```python
from build123d import *

# Parameters (mm, degrees)
SKETCH_1_R             = 16
EXTRUDE_1_DEPTH        = 12
SKETCH_2_R             = 13
EXTRUDE_2_DEPTH        = 2
SKETCH_3_R             = 12.25
EXTRUDE_4_DEPTH        = 11.2
SKETCH_4_R             = 1.5
EXTRUDE_5_DEPTH        = 2
SKETCH_21_W            = 0.599041837
SKETCH_21_H            = 5.051087673
CUT_EXTRUDE_2_DEPTH    = 5
HOLE_WIZARD_M3_1_D     = 2.5
HOLE_WIZARD_M3_1_DEPTH = 7.5
HOLE_WIZARD_M3_1_TIP   = 0.751075774
EXTRUDE_16_DEPTH       = 15


with BuildPart() as part:
    # 草图1 → 凸台-拉伸1 (new body)
    with BuildSketch(Plane.XY):
        Circle(SKETCH_1_R)
    extrude(amount=-EXTRUDE_1_DEPTH)

    # 草图2 → 凸台-拉伸2 (add)
    with BuildSketch(Plane(origin=(0, 0, -12), x_dir=(-1, 0, 0), z_dir=(0, 0, -1))):
        Circle(SKETCH_2_R)
    extrude(amount=EXTRUDE_2_DEPTH)

    # 草图3 → 凸台-拉伸4 (add)
    with BuildSketch(Plane(origin=(0, 0, -14), x_dir=(-1, 0, 0), z_dir=(0, 0, -1))):
        with Locations(Location((0, 0, 0), (0, 0, 180))):
            Circle(SKETCH_3_R)
    extrude(amount=EXTRUDE_4_DEPTH)

    # 草图4 → 凸台-拉伸5 (add)
    # profile 1 of 2: a face of its own
    with BuildSketch(Plane.XY):
        with BuildLine():
            Line((-4, 19.5), (-4, 15.491933385))
            ThreePointArc((-4, 15.491933385), (0, 16), (4, 15.491933385))
            Line((4, 15.491933385), (4, 19.5))
            ThreePointArc((4, 19.5), (0, 23.5), (-4, 19.5))
        make_face()
        with Locations((0, 19.5)):
            Circle(SKETCH_4_R, mode=Mode.SUBTRACT)
    # profile 2 of 2: a face of its own
    with BuildSketch(Plane.XY):
        with BuildLine():
            Line((-4, -15.491933385), (-4, -19.5))
            ThreePointArc((-4, -19.5), (0, -23.5), (4, -19.5))
            Line((4, -19.5), (4, -15.491933385))
            ThreePointArc((4, -15.491933385), (0, -16), (-4, -15.491933385))
        make_face()
        with Locations(Location((0, -19.5, 0), (0, 0, 180))):
            Circle(SKETCH_4_R, mode=Mode.SUBTRACT)
    extrude(amount=-EXTRUDE_5_DEPTH)

    # 草图17 → 旋转1 (revolve)
    with BuildSketch(Plane(origin=(0, 0, 0), x_dir=(1, 0, 0), z_dir=(0, 1, 0)), mode=Mode.PRIVATE) as revolve_1_sk:
        Polygon((8, -10.2), (8, 0), (3.5, 0), (3.5, -1.25), (4, -1.25), (4, -2.7), (5.5, -2.7), (5.5, -10.2), align=None)
    revolve(revolve_1_sk.sketch.rotate(Axis((8, 0, 10.2), (0, 0, -1)), 180), axis=Axis((8, 0, 10.2), (0, 0, -1)))

    # 草图21 → 切除-拉伸2 (cut)
    with BuildSketch(Plane.XY.offset(10.2)):
        with Locations((5.700479082, -0.105298995)):
            Rectangle(SKETCH_21_W, SKETCH_21_H)
        with Locations((10.299520919, -0.105298995)):
            Rectangle(SKETCH_21_W, SKETCH_21_H)
    extrude(amount=-CUT_EXTRUDE_2_DEPTH, mode=Mode.SUBTRACT)

    # M3 螺纹孔1
    with Locations(Plane.XY.offset(10.2)):
        with Locations((8, 0)):
            Hole(HOLE_WIZARD_M3_1_D / 2, depth=HOLE_WIZARD_M3_1_DEPTH)
            with Locations((0, 0, -(HOLE_WIZARD_M3_1_DEPTH + HOLE_WIZARD_M3_1_TIP / 2))):  # 118° drill point
                Cone(0, HOLE_WIZARD_M3_1_D / 2, HOLE_WIZARD_M3_1_TIP, mode=Mode.SUBTRACT)

    # 草图25 → 凸台-拉伸16 (add)
    with BuildSketch(Plane(origin=(0, 0, 0), x_dir=(0, 0, -1), z_dir=(1, 0, 0))):
        with BuildLine():
            Line((24.65972398, 2.283115818), (24.65972398, -2.515790041))
            ThreePointArc((24.65972398, -2.515790041), (23.758111364, -3.417402657), (22.856498748, -2.515790041))
            Line((22.856498748, -2.515790041), (22.856498748, 2.283115818))
            ThreePointArc((22.856498748, 2.283115818), (23.758111364, 3.184728434), (24.65972398, 2.283115818))
        make_face()
    extrude(amount=EXTRUDE_16_DEPTH)


solid = part.part
```
Source: CAD feature listing. Evaluate the final solid. Frame: model axes, mm. A direction names the side the tool comes from. Round coordinates to 2 decimals unless told otherwise and drop trailing zeros. Loops run counter-clockwise (first coordinate to the right, second up) from the corner with the lowest first, then second, coordinate; pieces in that order, holes last.
1. Section query C-C on x = -9. Output: boundary loops of the cut face in (y, z).
2. Mould query, pull axis Z, two halves, no side actions, for faces 4 (the cylindrical face through (0, -21, -1)), 5 (the flat face through (0, 0, 0)), 6 (the cylindrical face through (13.392, 3.185, -23.738)). Classes: released by +Z, released by -Z, zero draft, split by the parting line, or undercut.
3. Contact query for flat-ended pins moving along their axis: pin 1 (0.6 mm diameter, centred on x = 5.5, y = -0.5, fed in from +Z); pin 2 (0.5 mm diameter, centred on y = -1.5, z = -23.5, fed in from +X); pin 3 (1 mm diameter, centred on x = 6, z = -9.5, fed in from -Y) (3 decimals); pin 4 (2 mm diameter, centred on x = -9.5, y = 15.5, fed in from -Z). Output: stop coordinate, or through.
4. Section query B-B on z = 6.5. Output: boundary loops of the cut face in (x, y), and give its area (3 significant figures).
5. Ray query, L1, parallel to Y at x = 0, z = -0.5; L2, parallel to X at y = -19.5, z = -1.6; L3, parallel to X at y = 0, z = 8. Return the intervals inside material, ascending.
6. Access query for faces 1 (the cylindrical face through (13.359, -3.417, -23.778)), 2 (the flat face through (15, 0, -24)), 3 (the flat face through (4, -18, -1)). Directions: +Z, -Z, +X, -X, +Y, -Y. A direction counts if a zero-diameter tool reaches every point of the face in a straight line with its end or side. Return the directions, or none.
7. Section query D-D on z = -4.5. Output: boundary loops of the cut face in (x, y).
8. Section query A-A on x = 0. Output: boundary loops of the cut face in (y, z), and give its area (3 significant figures).
Answers below:
1. outline: (-13.23, -12) - (-9.38, -12) - (-9.38, -14) - (-8.31, -14) - (-8.31, -25.2) - (8.31, -25.2) - (8.31, -14) - (9.38, -14) - (9.38, -12) - (13.23, -12) - (13.23, 0) - (-13.23, 0) - close
2. face 4: zero draft
2. face 5: released by +Z
2. face 6: undercut
3. pin 1: stops at z = 5.2
3. pin 2: stops at x = 15
3. pin 3: stops at y = -15.025
3. pin 4: passes through
4. outline: (6, -1.5) arc R2.5 ccw to (10, -1.5) - (10, 1.5) arc R2.5 ccw to (6, 1.5) - close; hole circle Ø2.5 at (8, 0)
4. area: 12.7 mm2
5. L1: y = -23.5 to -21, -18 to 18, 21 to 23.5
5. L2: x = -4 to -1.5, 1.5 to 4
5. L3: x = 6 to 6.75, 9.25 to 10
6. face 1: +X, -Y
6. face 2: -Z, +X, +Y, -Y
6. face 3: +Z, -Z, +X, -Y
7. outline: circle Ø32 at (0, 0)
8. outline: (-23.5, -2) - (-21, -2) - (-21, 0) - (-23.5, 0) - close; (-18, -2) - (-16, -2) - (-16, -12) - (-13, -12) - (-13, -14) - (-12.25, -14) - (-12.25, -25.2) - (12.25, -25.2) - (12.25, -14) - (13, -14) - (13, -12) - (16, -12) - (16, -2) - (18, -2) - (18, 0) - (-18, 0) - close; (21, -2) - (23.5, -2) - (23.5, 0) - (21, 0) - close
8. area: 728 mm2
